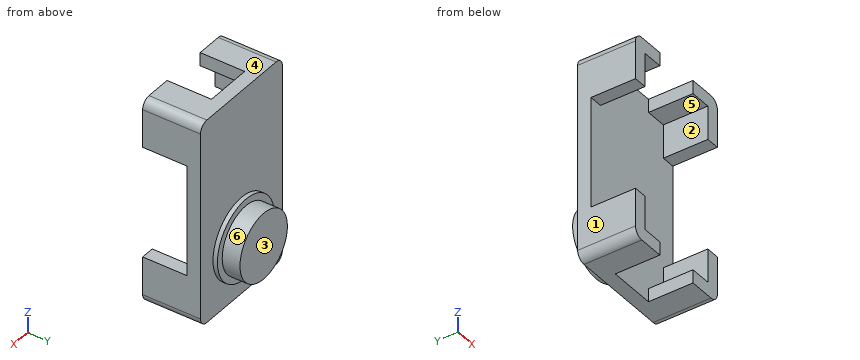
```python
from build123d import *

# Parameters (mm, degrees)
CROQUIS1_W              = 25.9
CROQUIS1_H              = 46.2
CROQUIS1_W_2            = 19.9
CROQUIS1_H_2            = 40.2
SALIENTE_EXTRUIR1_DEPTH = 10
CROQUIS2_W              = 25.9
CROQUIS2_H              = 46.2
SALIENTE_EXTRUIR2_DEPTH = 3
CROQUIS3_W              = 10.5
CROQUIS3_H              = 46.2
CORTAR_EXTRUIR1_DEPTH   = 17
CROQUIS4_W              = 25.9
CROQUIS4_H              = 25
CORTAR_EXTRUIR2_DEPTH   = 17
CROQUIS5_R              = 7.5
SALIENTE_EXTRUIR3_DEPTH = 5
CROQUIS6_R              = 9
SALIENTE_EXTRUIR4_DEPTH = 1
REDONDEO1_R             = 2


with BuildPart() as part:
    # Croquis1 → Saliente-Extruir1 (new body)
    with BuildSketch(Plane(origin=(0, 0, 0), x_dir=(1, 0, 0), z_dir=(0, 1, 0))):
        Rectangle(CROQUIS1_W, CROQUIS1_H)
        Rectangle(CROQUIS1_W_2, CROQUIS1_H_2, mode=Mode.SUBTRACT)
    extrude(amount=SALIENTE_EXTRUIR1_DEPTH)

    # Croquis2 → Saliente-Extruir2 (add)
    with BuildSketch(Plane(origin=(0, 10, 0), x_dir=(1, 0, 0), z_dir=(0, 1, 0))):
        Rectangle(CROQUIS2_W, CROQUIS2_H)
    extrude(amount=SALIENTE_EXTRUIR2_DEPTH)

    # Croquis3 → Cortar-Extruir1 (cut)
    with BuildSketch(Plane.XZ.offset(-10)):
        Rectangle(CROQUIS3_W, CROQUIS3_H)
    extrude(amount=CORTAR_EXTRUIR1_DEPTH, mode=Mode.SUBTRACT)

    # Croquis4 → Cortar-Extruir2 (cut)
    with BuildSketch(Plane.XZ.offset(-10)):
        Rectangle(CROQUIS4_W, CROQUIS4_H)
    extrude(amount=CORTAR_EXTRUIR2_DEPTH, mode=Mode.SUBTRACT)

    # Croquis5 → Saliente-Extruir3 (add)
    with BuildSketch(Plane(origin=(0, 13, 0), x_dir=(1, 0, 0), z_dir=(0, 1, 0))):
        with Locations((0, 10.15)):
            Circle(CROQUIS5_R)
    extrude(amount=SALIENTE_EXTRUIR3_DEPTH)

    # Croquis6 → Saliente-Extruir4 (add)
    with BuildSketch(Plane(origin=(0, 13, 0), x_dir=(1, 0, 0), z_dir=(0, 1, 0))):
        with Locations((0, 10.15)):
            Circle(CROQUIS6_R)
    extrude(amount=SALIENTE_EXTRUIR4_DEPTH)

    # Redondeo1
    redondeo1_edges = [part.edges().sort_by_distance(p)[0] for p in [
        (12.95, 6.5, 23.1),
        (-12.95, 6.5, 23.1),
        (-12.95, 6.5, -23.1),
        (12.95, 6.5, -23.1),
    ]]
    fillet(redondeo1_edges, radius=REDONDEO1_R)


solid = part.part
```
Part model, mm, in its own coordinate system. Face numbers are marked on the shaded views. A direction names the side the tool comes from. Round coordinates to 2 decimals unless told otherwise and drop trailing zeros. Loops run counter-clockwise (first coordinate to the right, second up) from the corner with the lowest first, then second, coordinate; pieces in that order, holes last. Notation, with made-up numbers: (-20, -27.5) -> (-16, -27.5) arc R16 cw to (-16, -4.5) -> close; hole circle Ø10 at (-4, -10). An arc over 180 degrees is marked (long way). Use one line per item in the form item = value. Start each with the question number.
Item 1: Band-saw the part on C-C (z = -10.15). List the corners of the cut face in (x, y).
Item 2: Drill centre lines: line 1 along X through (y, z) = (2, 13); line 2 along Z through (x, y) = (8, 6); line 3 along Z through (x, y) = (10.5, 7.25). Where is each one in solid material? Low to high.
Item 3: Band-saw the part on B-B (x = 0). List the corners of the cut face in (y, z).
Item 4: Tool access for the marked faces 4, 5 and 6: list every direction of +Z, -Z, +X, -X, +Y, -Y with a clear straight run to the whole face (end or side of a thin tool).
Item 5: Two-plate mould, pull along X, no slides. Class the marked faces 1, 2 and 3: released by +X, released by -X, zero draft, split by the parting line, or undercut.
Item 6: Drop flat-ended pins along their axis: pin 1 Ø6 at (x, y) = (-3, 3.5) entering from +Z; pin 2 Ø0.9 at (y, z) = (6, 22) entering from -X; pin 3 Ø10 at (x, z) = (-10, -0.5) entering from +Y. Give the stop position or say it passes through.
Item 7: Band-saw the part on A-A (y = 4.5). List the corners of the cut face in (x, z).
Data:
q1.outline = (-12.95, 10) -> (12.95, 10) -> (12.95, 13) -> (9, 13) -> (9, 14) -> (7.5, 14) -> (7.5, 18) -> (-7.5, 18) -> (-7.5, 14) -> (-9, 14) -> (-9, 13) -> (-12.95, 13) -> close
q2.line_1 = -12.95 to -9.95, 9.95 to 12.95
q2.line_2 = -23.1 to -20.1, 20.1 to 23.1
q2.line_3 = -23.1 to -12.5, 12.5 to 23.1
q3.outline = (10, -23.1) -> (13, -23.1) -> (13, -19.15) -> (14, -19.15) -> (14, -17.65) -> (18, -17.65) -> (18, -2.65) -> (14, -2.65) -> (14, -1.15) -> (13, -1.15) -> (13, 23.1) -> (10, 23.1) -> close
q4.face_4 = +Z, +X, -X, +Y, -Y
q4.face_5 = -Y
q4.face_6 = +Y
q5.face_1 = released by -X
q5.face_2 = undercut
q5.face_3 = zero draft
q6.pin_1 = 23.1
q6.pin_2 = -12.9
q6.pin_3 = 14
q7.outline = (-12.95, -21.1) arc R2 ccw to (-10.95, -23.1) -> (-5.25, -23.1) -> (-5.25, -20.1) -> (-9.95, -20.1) -> (-9.95, -12.5) -> (-12.95, -12.5) -> close; (-12.95, 12.5) -> (-9.95, 12.5) -> (-9.95, 20.1) -> (-5.25, 20.1) -> (-5.25, 23.1) -> (-10.95, 23.1) arc R2 ccw to (-12.95, 21.1) -> close; (5.25, -23.1) -> (10.95, -23.1) arc R2 ccw to (12.95, -21.1) -> (12.95, -12.5) -> (9.95, -12.5) -> (9.95, -20.1) -> (5.25, -20.1) -> close; (5.25, 20.1) -> (9.95, 20.1) -> (9.95, 12.5) -> (12.95, 12.5) -> (12.95, 21.1) arc R2 ccw to (10.95, 23.1) -> (5.25, 23.1) -> close
